Can you work these out from the model? Positions are in its coordinate system, mm. Give positions to 0.01 mm unless a question says otherwise; leave off trailing zeros.
1. If I drill on probe 1 along X at (y, z) = (15, 792); probe 2 along Y at (x, z) = (-15, 767.5); probe 3 along Y at (x, z) = (-25, 790.5), over which ranges is the centre line in solid material (lowest first)?
2. Suppose I cut it at A-A (z = 579). Give the number of separate pieces and of enclosed holes in the cut face, and give its area (3 significant figures).
3. I'm going to push flat-ended pins straight in: pin 1 (8 mm diameter, centred on y = 14, z = 285.5, fed in from -X); pin 2 (12 mm diameter, centred on x = -8.5, y = -10.5, fed in from -Z). Where does each tip first touch, or does it pass through?
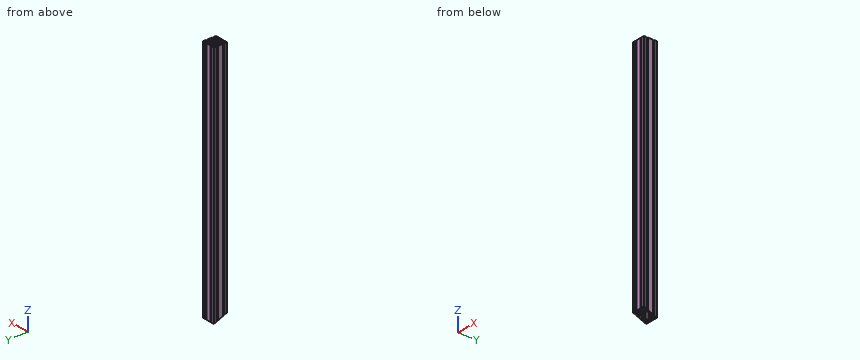
```python
from build123d import *

# Parameters (mm, degrees)
F0_R          = 3
F0_R_2        = 2.5
F1_DEPTH      = 1100.6
F2_R          = 2
F3_R          = 7
F5_DEPTH      = 30
F5_DEPTH_BACK = 30


# Not quite as in the source:
# - a feature names something its author has since deleted; it is built from what else it names


with BuildPart() as f1:
    # F0 (on Top) → F1 (new body)
    with BuildSketch(Plane.XY):
        with BuildLine():
            Line((18.15, -30), (30, -30))
            Line((30, -30), (30, -18.15))
            Line((30, -18.15), (27.5, -18.15))
            Line((27.5, -18.15), (27.5, -20.15))
            Line((27.5, -20.15), (21.5477069044, -20.15))
            ThreePointArc((21.5477069044, -20.15), (19.5, -15), (21.5477069044, -9.85))
            Line((21.5477069044, -9.85), (27.5, -9.85))
            Line((27.5, -9.85), (27.5, -11.85))
            Line((27.5, -11.85), (30, -11.85))
            Line((30, -11.85), (30, 11.85))
            Line((30, 11.85), (27.5, 11.85))
            Line((27.5, 11.85), (27.5, 9.85))
            Line((27.5, 9.85), (21.5477069044, 9.85))
            ThreePointArc((21.5477069044, 9.85), (19.5, 15), (21.5477069044, 20.15))
            Line((21.5477069044, 20.15), (27.5, 20.15))
            Line((27.5, 20.15), (27.5, 18.15))
            Line((27.5, 18.15), (30, 18.15))
            Line((30, 18.15), (30, 30))
            Line((30, 30), (18.15, 30))
            Line((18.15, 30), (18.15, 27.5))
            Line((18.15, 27.5), (20.15, 27.5))
            Line((20.15, 27.5), (20.15, 21.5477069044))
            ThreePointArc((20.15, 21.5477069044), (15, 19.5), (9.85, 21.5477069044))
            Line((9.85, 21.5477069044), (9.85, 27.5))
            Line((9.85, 27.5), (11.85, 27.5))
            Line((11.85, 27.5), (11.85, 30))
            Line((11.85, 30), (-11.85, 30))
            Line((-11.85, 30), (-11.85, 27.5))
            Line((-11.85, 27.5), (-9.85, 27.5))
            Line((-9.85, 27.5), (-9.85, 21.5477069044))
            ThreePointArc((-9.85, 21.5477069044), (-15, 19.5), (-20.15, 21.5477069044))
            Line((-20.15, 21.5477069044), (-20.15, 27.5))
            Line((-20.15, 27.5), (-18.15, 27.5))
            Line((-18.15, 27.5), (-18.15, 30))
            Line((-18.15, 30), (-30, 30))
            Line((-30, 30), (-30, 18.15))
            Line((-30, 18.15), (-27.5, 18.15))
            Line((-27.5, 18.15), (-27.5, 20.15))
            Line((-27.5, 20.15), (-21.5477069044, 20.15))
            ThreePointArc((-21.5477069044, 20.15), (-19.5, 15), (-21.5477069044, 9.85))
            Line((-21.5477069044, 9.85), (-27.5, 9.85))
            Line((-27.5, 9.85), (-27.5, 11.85))
            Line((-27.5, 11.85), (-30, 11.85))
            Line((-30, 11.85), (-30, -11.85))
            Line((-30, -11.85), (-27.5, -11.85))
            Line((-27.5, -11.85), (-27.5, -9.85))
            Line((-27.5, -9.85), (-21.5477069044, -9.85))
            ThreePointArc((-21.5477069044, -9.85), (-19.5, -15), (-21.5477069044, -20.15))
            Line((-21.5477069044, -20.15), (-27.5, -20.15))
            Line((-27.5, -20.15), (-27.5, -18.15))
            Line((-27.5, -18.15), (-30, -18.15))
            Line((-30, -18.15), (-30, -30))
            Line((-30, -30), (-18.15, -30))
            Line((-18.15, -30), (-18.15, -27.5))
            Line((-18.15, -27.5), (-20.15, -27.5))
            Line((-20.15, -27.5), (-20.15, -21.5477069044))
            ThreePointArc((-20.15, -21.5477069044), (-15, -19.5), (-9.85, -21.5477069044))
            Line((-9.85, -21.5477069044), (-9.85, -27.5))
            Line((-9.85, -27.5), (-11.85, -27.5))
            Line((-11.85, -27.5), (-11.85, -30))
            Line((-11.85, -30), (11.85, -30))
            Line((11.85, -30), (11.85, -27.5))
            Line((11.85, -27.5), (9.85, -27.5))
            Line((9.85, -27.5), (9.85, -21.5477069044))
            ThreePointArc((9.85, -21.5477069044), (15, -19.5), (20.15, -21.5477069044))
            Line((20.15, -21.5477069044), (20.15, -27.5))
            Line((20.15, -27.5), (18.15, -27.5))
            Line((18.15, -27.5), (18.15, -30))
        make_face()
        with Locations((-25, -25)):
            Circle(F0_R, mode=Mode.SUBTRACT)
        with Locations((-15, -15)):
            Circle(F0_R_2, mode=Mode.SUBTRACT)
        with Locations((25, -25)):
            Circle(F0_R, mode=Mode.SUBTRACT)
        with Locations((15, -15)):
            Circle(F0_R_2, mode=Mode.SUBTRACT)
        with Locations((-25, 25)):
            Circle(F0_R, mode=Mode.SUBTRACT)
        with Locations((-15, 15)):
            Circle(F0_R_2, mode=Mode.SUBTRACT)
        Polygon((-7, 22), (-7, 27.5), (0, 27.5), (7, 27.5), (7, 22), (10, 16), (10, 10), (16, 10), (22, 7), (27.5, 7), (27.5, 0), (27.5, -7), (22, -7), (16, -10), (10, -10), (10, -16), (7, -22), (7, -27.5), (0, -27.5), (-7, -27.5), (-7, -22), (-10, -16), (-10, -10), (-16, -10), (-22, -7), (-27.5, -7), (-27.5, 0), (-27.5, 7), (-22, 7), (-16, 10), (-10, 10), (-10, 16), align=None, mode=Mode.SUBTRACT)
        with Locations((15, 15)):
            Circle(F0_R_2, mode=Mode.SUBTRACT)
        with Locations((25, 25)):
            Circle(F0_R, mode=Mode.SUBTRACT)
    extrude(amount=F1_DEPTH)

    # F2
    f2_edges = [f1.edges().sort_by_distance(p)[0] for p in [
        (-7, 27.5, 550.3),
        (7, 27.5, 550.3),
    ]]
    fillet(f2_edges, radius=F2_R)

    # F3
    f3_edges = [f1.edges().sort_by_distance(p)[0] for p in [
        (-10, 16, 550.3),
        (10, 16, 550.3),
    ]]
    fillet(f3_edges, radius=F3_R)

    # F4 (on Right) → F5 (cut, two sides)
    with BuildSketch(Plane.YZ) as f5_sk:
        Polygon((-153.0130330148, 75.8064803658), (-200.6900714338, -39.2960723993), (-17.6770384191, -115.1025527651), (30, 0), align=None)
    extrude(amount=F5_DEPTH, mode=Mode.SUBTRACT)
    extrude(f5_sk.sketch, amount=-F5_DEPTH_BACK, mode=Mode.SUBTRACT)


solid = f1.part
```
Checks:
1. probe 1: x = -19.5 to -17.5, -12.5 to -9.97, 9.97 to 12.5, 17.5 to 19.5
1. probe 2: y = -19.5 to -17.5, -12.5 to -10, 10 to 12.5, 17.5 to 19.5
1. probe 3: y = -30 to -28, -22 to -20.15, -9.85 to -7, 7 to 9.85, 20.15 to 22, 28 to 30
2. separate pieces: 1
2. enclosed holes: 9
2. area: 1,080 mm2
3. pin 1: stops at x = -30
3. pin 2: stops at z = 16.57
